Read the model definition and answer for the solid it produces. Units are mm, in the model's axes. Face numbers are marked on the shaded views. A direction names the side the tool comes from. Give positions to 0.01 mm unless a question says otherwise; leave off trailing zeros. Write each loop counter-clockwise with the first axis right and the second up, starting at its lowest first coordinate (ties: lowest second). Pieces come first, ordered by that corner, then holes.
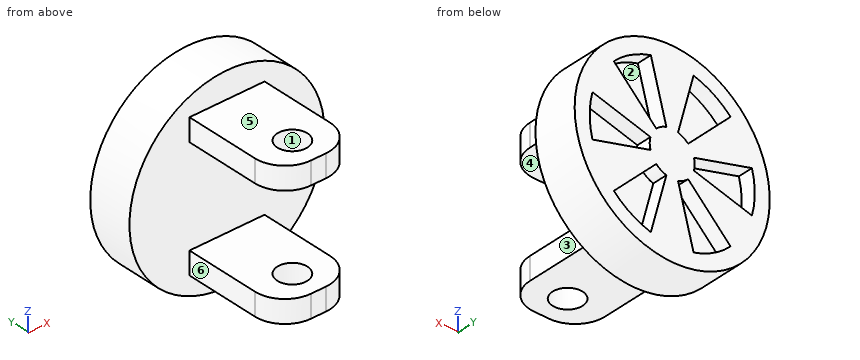
```python
from build123d import *

# Parameters (mm, degrees)
SKETCH_1_R          = 65
EXTRUDE_1_DEPTH     = 30
SKETCH_2_W          = 50
SKETCH_2_H          = 15
EXTRUDE_2_DEPTH     = 70
FILLET_2_R          = 20
SKETCH_3_R          = 10
CUT_EXTRUDE_1_DEPTH = 113.5
CUT_EXTRUDE_2_DEPTH = 10


with BuildPart() as part:
    # 草图1 → 凸台-拉伸1 (new body)
    with BuildSketch(Plane(origin=(0, 0, 0), x_dir=(1, 0, 0), z_dir=(0, 1, 0))):
        Circle(SKETCH_1_R)
    extrude(amount=EXTRUDE_1_DEPTH)

    # 草图2 → 凸台-拉伸2 (add)
    with BuildSketch(Plane.XZ):
        with Locations((0, 40)):
            Rectangle(SKETCH_2_W, SKETCH_2_H)
        with Locations((0, -40)):
            Rectangle(SKETCH_2_W, SKETCH_2_H)
    extrude(amount=EXTRUDE_2_DEPTH)

    # 圆角2
    fillet_2_edges = [part.edges().sort_by_distance(p)[0] for p in [
        (25, -70, 40),
        (-25, -70, 40),
        (-25, -70, -40),
        (25, -70, -40),
    ]]
    fillet(fillet_2_edges, radius=FILLET_2_R)

    # 草图3 → 切除-拉伸1 (cut, through all)
    with BuildSketch(Plane.XY.offset(47.5)):
        with Locations((0, -50)):
            Circle(SKETCH_3_R)
    extrude(amount=-CUT_EXTRUDE_1_DEPTH, mode=Mode.SUBTRACT)

    # 草图7 → 切除-拉伸2 (cut)
    with BuildSketch(Plane(origin=(0, 30, 0), x_dir=(1, 0, 0), z_dir=(0, 1, 0))):
        with BuildLine():
            Line((14.488887394, 3.882285677), (53.125920446, 14.235047481))
            ThreePointArc((53.125920446, 14.235047481), (55, 0), (53.125920446, -14.235047481))
            Line((53.125920446, -14.235047481), (14.488887394, -3.882285677))
            ThreePointArc((14.488887394, -3.882285677), (15, 0), (14.488887394, 3.882285677))
        make_face()
        with BuildLine():
            Line((10.606601718, -10.606601718), (38.890872965, -38.890872965))
            ThreePointArc((38.890872965, -38.890872965), (27.5, -47.631397208), (14.235047481, -53.125920446))
            Line((14.235047481, -53.125920446), (3.882285677, -14.488887394))
            ThreePointArc((3.882285677, -14.488887394), (7.5, -12.990381057), (10.606601718, -10.606601718))
        make_face()
        with BuildLine():
            Line((-3.882285677, -14.488887394), (-14.235047481, -53.125920446))
            ThreePointArc((-14.235047481, -53.125920446), (-27.5, -47.631397208), (-38.890872965, -38.890872965))
            Line((-38.890872965, -38.890872965), (-10.606601718, -10.606601718))
            ThreePointArc((-10.606601718, -10.606601718), (-7.5, -12.990381057), (-3.882285677, -14.488887394))
        make_face()
        with BuildLine():
            Line((-14.488887394, -3.882285677), (-53.125920446, -14.235047481))
            ThreePointArc((-53.125920446, -14.235047481), (-55, 0), (-53.125920446, 14.235047481))
            Line((-53.125920446, 14.235047481), (-14.488887394, 3.882285677))
            ThreePointArc((-14.488887394, 3.882285677), (-15, 0), (-14.488887394, -3.882285677))
        make_face()
        with BuildLine():
            Line((-10.606601718, 10.606601718), (-38.890872965, 38.890872965))
            ThreePointArc((-38.890872965, 38.890872965), (-27.5, 47.631397208), (-14.235047481, 53.125920446))
            Line((-14.235047481, 53.125920446), (-3.882285677, 14.488887394))
            ThreePointArc((-3.882285677, 14.488887394), (-7.5, 12.990381057), (-10.606601718, 10.606601718))
        make_face()
        with BuildLine():
            Line((3.882285677, 14.488887394), (14.235047481, 53.125920446))
            ThreePointArc((14.235047481, 53.125920446), (27.5, 47.631397208), (38.890872965, 38.890872965))
            Line((38.890872965, 38.890872965), (10.606601718, 10.606601718))
            ThreePointArc((10.606601718, 10.606601718), (7.5, 12.990381057), (3.882285677, 14.488887394))
        make_face()
    extrude(amount=-CUT_EXTRUDE_2_DEPTH, mode=Mode.SUBTRACT)


solid = part.part
```
Item 1: Section A-A (y = -14) is taken. Write down the section's boundary in (x, z).
Result set:
outline: (-25, -47.5) - (25, -47.5) - (25, -32.5) - (-25, -32.5) - close; (-25, 32.5) - (25, 32.5) - (25, 47.5) - (-25, 47.5) - close
Item 2: Section D-D (z = -42.5) is taken. Write down the section's boundary in (x, y), and give its area (3 significant figures).
Result set:
outline: (-49.18, 0) - (-25, 0) - (-25, -50) arc R20 ccw to (-5, -70) - (5, -70) arc R20 ccw to (25, -50) - (25, 0) - (49.18, 0) - (49.18, 30) - (34.91, 30) - (34.91, 20) - (11.39, 20) - (11.39, 30) - (-11.39, 30) - (-11.39, 20) - (-34.91, 20) - (-34.91, 30) - (-49.18, 30) - close; hole circle Ø20 at (0, -50)
area: 5,490 mm2
Item 3: Determine the mould class of the marked faces 1, 2 and 3 for opening direction Y: pulls with the +Y half, pulls with the -Y half, needs draft (parallel to the pull), parting line crosses it, or undercut.
Result set:
face 1: undercut
face 2: pulls with the +Y half
face 3: needs draft
Item 4: Which of the six approach directions +Z, -Z, +X, -X, +Y, -Y give full straight-line access (tool end or side, diameter ignored) to the marked faces 4, 5 and 6?
Result set:
face 4: +X, -X, -Y
face 5: +Z, +X, -X, -Y
face 6: +Z, -Z, -X, -Y
Item 5: Each of these flat-tipped pins is pushed along its axis until it touches: pin 1 Ø15 at (x, y) = (0, -24.5) entering from -Z; pin 2 Ø5 at (x, y) = (20, 4.5) entering from -Z; pin 3 Ø2 at (y, z) = (20, 17) entering from -X; pin 4 Ø10.5 at (x, z) = (13, 33.5) entering from +Y. Where does it stop, or does it pass through?
Result set:
pin 1: stops at z = -47.5
pin 2: stops at z = -62.6
pin 3: stops at x = -63
pin 4: stops at y = 30
Item 6: Section C-C (z = 0) is taken. Write down the section's boundary in (x, y).
Result set:
outline: (-65, 0) - (65, 0) - (65, 30) - (55, 30) - (55, 20) - (15, 20) - (15, 30) - (-15, 30) - (-15, 20) - (-55, 20) - (-55, 30) - (-65, 30) - close
Item 7: Find the intervals of material crossed by line 1 along Z through (x, y) = (1.5, -26); line 2 along Y through (x, z) = (0, 37.5); line 3 along Z through (x, y) = (19, 25), in increasing order.
Result set:
line 1: z = -47.5 to -32.5, 32.5 to 47.5
line 2: y = -70 to -60, -40 to 30
line 3: z = -62.16 to -51.61, -19 to -5.09, 5.09 to 19, 51.61 to 62.16
Item 8: Section B-B (x = 0) is taken. Write down the section's boundary in (y, z), and give its area (3 significant figures).
Result set:
outline: (-70, -47.5) - (-60, -47.5) - (-60, -32.5) - (-70, -32.5) - close; (-70, 32.5) - (-60, 32.5) - (-60, 47.5) - (-70, 47.5) - close; (-40, -47.5) - (0, -47.5) - (0, -65) - (30, -65) - (30, 65) - (0, 65) - (0, 47.5) - (-40, 47.5) - (-40, 32.5) - (0, 32.5) - (0, -32.5) - (-40, -32.5) - close
area: 5,400 mm2
